Verification items for this drawing (mm, ordinates from the low corner). Round coordinates to 2 decimals unless told otherwise and drop trailing zeros. Order: outer loops, then holes, each group sorted by start corner. A loop starts at its lowest first (then second) coordinate and runs counter-clockwise, first axis right, second up. Notation, with made-up numbers: M 8,71.25 L 67,71.25 A31 ccw 67,96.25 Z; hole C -27.5,-22 d4. An arc over 180 degrees is marked long. One line per item, written item: value. Start each with the question number.
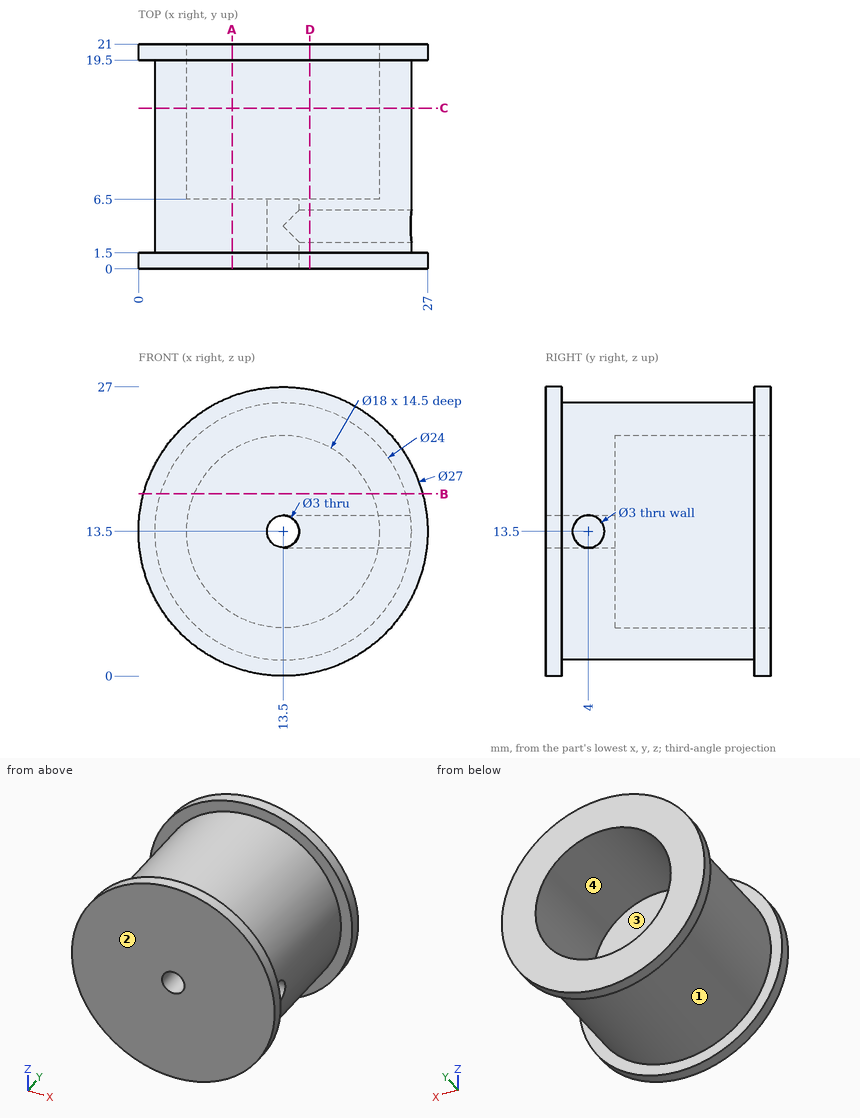
1. Section check C-C (y = 15). Record the cut outline in (x, z).
2. Section check A-A (x = 8.75). Record the cut outline in (y, z).
3. Section check B-B (z = 17). Record the cut outline in (x, y), and give its area (3 significant figures).
4. Scan lines: line 1 along Y through (x, z) = (16.25, 13.5); line 2 along Z through (x, y) = (13.5, 2); line 3 along Y through (x, z) = (7.25, 25.25). Record each from-to range of solid material in increasing order.
5. Draft check along Y on the marked faces 1, 2, 3 and 4. Enter one of: released by +Y, released by -Y, zero draft, split by the parting line, or undercut.
6. Depth check by flat-ended pin: pin 1 (3 mm diameter, centred on x = 13, z = 20.5, fed in from +Y); pin 2 (1.8 mm diameter, centred on x = 13.5, z = 13.5, fed in from -Y); pin 3 (1 mm diameter, centred on y = 4.5, z = 8.5, fed in from -X); pin 4 (3.5 mm diameter, centred on y = 4, z = 13.5, fed in from +X). Enter the tip coordinate at first touch or a pass-through.
7. Section check D-D (x = 16). Record the cut outline in (y, z).
Geometry check:
1. outline: C 13.5,13.5 d24; hole C 13.5,13.5 d18
2. outline: M 0,0.86 L 1.5,0.86 L 1.5,2.48 L 19.5,2.48 L 19.5,0.86 L 21,0.86 L 21,5.86 L 6.5,5.86 L 6.5,21.14 L 21,21.14 L 21,26.14 L 19.5,26.14 L 19.5,24.52 L 1.5,24.52 L 1.5,26.14 L 0,26.14 Z
3. outline: M 0.46,0 L 26.54,0 L 26.54,1.5 L 24.98,1.5 L 24.98,19.5 L 26.54,19.5 L 26.54,21 L 21.79,21 L 21.79,6.5 L 5.21,6.5 L 5.21,21 L 0.46,21 L 0.46,19.5 L 2.02,19.5 L 2.02,1.5 L 0.46,1.5 Z
3. area: 251 mm²
4. line 1: y = 0 to 2.5, 5.5 to 6.5
4. line 2: z = 1.5 to 12, 15 to 25.5
4. line 3: y = 0 to 1.5, 19.5 to 21
5. face 1: undercut
5. face 2: released by -Y
5. face 3: released by +Y
5. face 4: zero draft
6. pin 1: stops at y = 6.5
6. pin 2: passes through
6. pin 3: stops at x = 2.38
6. pin 4: stops at x = 25.5
7. outline: M 0,0.23 L 1.5,0.23 L 1.5,1.76 L 19.5,1.76 L 19.5,0.23 L 21,0.23 L 21,4.85 L 6.5,4.85 L 6.5,22.15 L 21,22.15 L 21,26.77 L 19.5,26.77 L 19.5,25.24 L 1.5,25.24 L 1.5,26.77 L 0,26.77 Z; hole C 4,13.5 d3
